Design review of the part built by this model. Coordinates are the model's own, in mm. Round coordinates to 2 decimals unless told otherwise and drop trailing zeros. Loops run counter-clockwise (first coordinate to the right, second up) from the corner with the lowest first, then second, coordinate; pieces in that order, holes last. Notation, with made-up numbers: M 68.25,35 L 73.25,35 A21 ccw 73.25,74 Z; hole C 54,-31 d10. An arc over 180 degrees is marked long. Use a Markdown table: item, result.
from build123d import *

# Parameters (mm, degrees)
BASE_DEPTH              = 3
CONG_1_R                = 3
ESQUISSE20_R            = 3
PERCAGE_PROFIL_S_DEPTH  = 383.50448595
ESQUISSE21_R            = 1.65
PERCAGE_LIDAR_DEPTH     = 383.50448595
ESQUISSE22_R            = 11.25
ENL_V_MAT_EXTRU_3_DEPTH = 383.50448595
ESQUISSE23_R            = 7
ENL_V_MAT_EXTRU_4_DEPTH = 383.50448595


with BuildPart() as part:
    # Esquisse1 → Base (new body)
    with BuildSketch(Plane.XY):
        Polygon((0, 0), (-200, 0), (-224.748737342, 24.748737342), (-224.748737342, 284.748737342), (-200, 309.497474683), (0, 309.497474683), (24.748737342, 284.748737342), (24.748737342, 24.748737342), align=None)
    extrude(amount=BASE_DEPTH)

    # Congé1
    cong_1_edges = [part.edges().sort_by_distance(p)[0] for p in [
        (0, 0, 1.5),
        (-200, 0, 1.5),
        (-224.748737342, 24.748737342, 1.5),
        (-224.748737342, 284.748737342, 1.5),
        (-200, 309.497474683, 1.5),
        (0, 309.497474683, 1.5),
        (24.748737342, 284.748737342, 1.5),
        (24.748737342, 24.748737342, 1.5),
    ]]
    fillet(cong_1_edges, radius=CONG_1_R)

    # Esquisse20 → Percage Profilés (cut, through all)
    with BuildSketch(Plane(origin=(0, 0, 0), x_dir=(-1, 0, 0), z_dir=(0, 0, -1))):
        with Locations((35, 286.497474683)):
            Circle(ESQUISSE20_R)
        with Locations(Location((165, 286.497474683, 0), (0, 0, 180))):
            Circle(ESQUISSE20_R)
        with Locations((165, 23)):
            Circle(ESQUISSE20_R)
        with Locations(Location((35, 23, 0), (0, 0, 180))):
            Circle(ESQUISSE20_R)
    extrude(amount=-PERCAGE_PROFIL_S_DEPTH, mode=Mode.SUBTRACT)

    # Esquisse21 → Percage Lidar (cut, through all)
    with BuildSketch(Plane(origin=(0, 0, 0), x_dir=(-1, 0, 0), z_dir=(0, 0, -1))):
        with Locations((61, 154.748737342)):
            Circle(ESQUISSE21_R)
        with Locations((100, 115.748737342)):
            Circle(ESQUISSE21_R)
    extrude(amount=-PERCAGE_LIDAR_DEPTH, mode=Mode.SUBTRACT)

    # Esquisse22 → Enlèv. mat.-Extru.3 (cut, through all)
    with BuildSketch(Plane(origin=(0, 0, 0), x_dir=(-1, 0, 0), z_dir=(0, 0, -1))):
        with Locations((68.560025138, 266.317142531)):
            Circle(ESQUISSE22_R)
    extrude(amount=-ENL_V_MAT_EXTRU_3_DEPTH, mode=Mode.SUBTRACT)

    # Esquisse23 → Enlèv. mat.-Extru.4 (cut, through all)
    with BuildSketch(Plane(origin=(0, 0, 0), x_dir=(-1, 0, 0), z_dir=(0, 0, -1))):
        with Locations((137.282259715, 262.406498542)):
            Circle(ESQUISSE23_R)
    extrude(amount=-ENL_V_MAT_EXTRU_4_DEPTH, mode=Mode.SUBTRACT)


solid = part.part
1. Take a section at A-A on x = -136.5. Give the boundary of the cut face in (y, z).
Check values:
| item | result |
|---|---|
| outline | M 0,0 L 255.45,0 L 255.45,3 L 0,3 Z; M 269.36,0 L 309.5,0 L 309.5,3 L 269.36,3 Z |
2. Wall thickness on line 1 along Y through (x, z) = (-35, 1.1); line 2 along Y through (x, z) = (-61, 0.95); line 3 along Y through (x, z) = (-100, 0.85): over which ranges is each line inside the solid? List them lowest first. Write a range as from..to.
Check values:
| item | result |
|---|---|
| line 1 | y = 0..20, 26..283.5, 289.5..309.5 |
| line 2 | y = 0..153.1, 156.4..257.99, 274.65..309.5 |
| line 3 | y = 0..114.1, 117.4..309.5 |
3. Take a section at B-B on z = 0.5. Count the separate pieces of the cut face and the enclosed holes in it, and give its area (3 significant figures).
Check values:
| item | result |
|---|---|
| separate pieces | 1 |
| enclosed holes | 8 |
| area | 75,300 mm² |
4. The part is to be moulded in two halves that separate along X. For faces 1 (the face through (-38, 23, 1)), 2 (the face through (-212, 12, 1)), 3 (the face through (-163.62, 289.16, 1.48)), 4 (the face through (12.2, 297.3, 1.5)), say which applies: pulls with the +X half, pulls with the -X half, needs draft (parallel to the pull), parting line crosses it, or undercut.
Check values:
| item | result |
|---|---|
| face 1 | undercut |
| face 2 | pulls with the -X half |
| face 3 | undercut |
| face 4 | pulls with the +X half |
